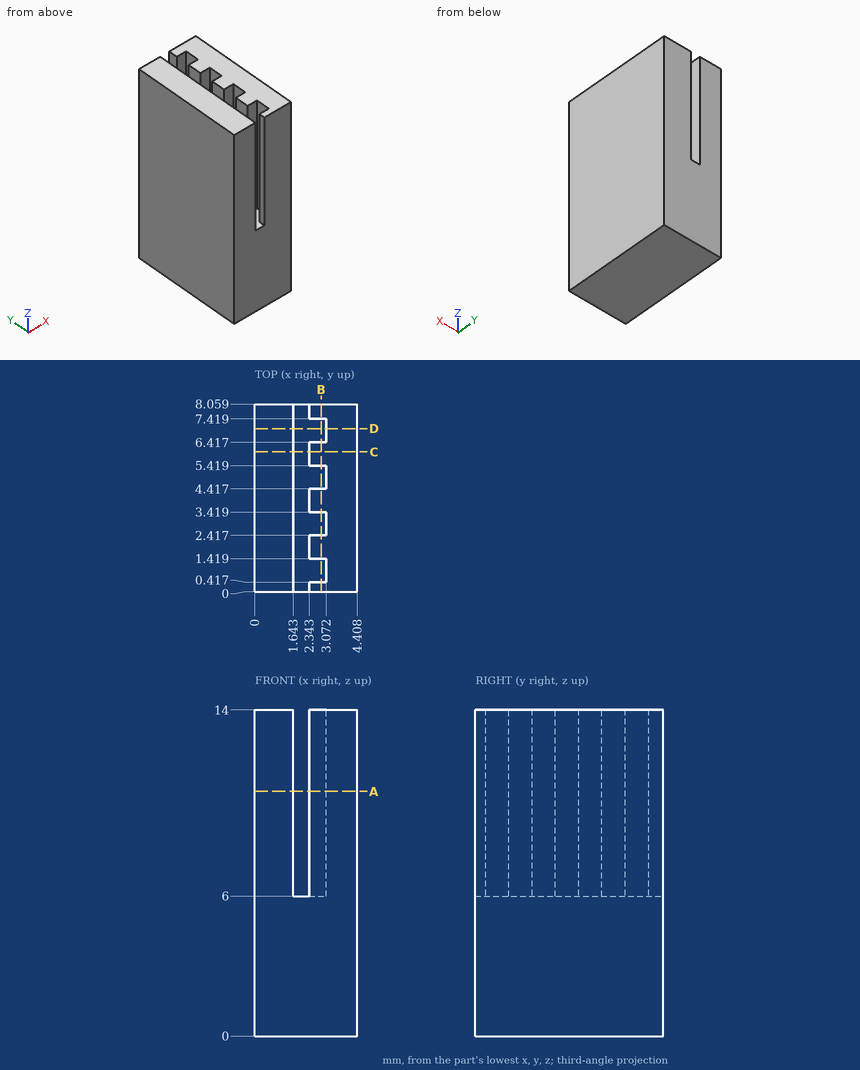
Geometry check sheet. Reference: drawing and pictorial views, mm from the part's lowest x, y, z. Round coordinates to 2 decimals unless told otherwise and drop trailing zeros. Write each loop counter-clockwise with the first axis right and the second up, starting at its lowest first coordinate (ties: lowest second). Pieces come first, ordered by that corner, then holes. Notation, with made-up numbers: (-19.5, 77) -> (12.5, 77) arc R24 ccw to (12.5, 114) -> close; hole circle Ø8 at (-18.75, -36.75). An arc over 180 degrees is marked (long way). Put each result on its own line as item: value.
1) Cross-section at D-D, the plane y = 7. Enter the section's corners in (x, z).
Recorded:
outline: (0, 0) -> (4.41, 0) -> (4.41, 14) -> (3.07, 14) -> (3.07, 6) -> (1.64, 6) -> (1.64, 14) -> (0, 14) -> close
2) Cross-section at B-B, the plane x = 2.85. Enter the section's corners in (y, z).
Recorded:
outline: (0, 0) -> (8.06, 0) -> (8.06, 14) -> (7.42, 14) -> (7.42, 6) -> (6.42, 6) -> (6.42, 14) -> (5.42, 14) -> (5.42, 6) -> (4.42, 6) -> (4.42, 14) -> (3.42, 14) -> (3.42, 6) -> (2.42, 6) -> (2.42, 14) -> (1.42, 14) -> (1.42, 6) -> (0.42, 6) -> (0.42, 14) -> (0, 14) -> close
3) Cross-section at A-A, the plane z = 10.5. Enter the section's corners in (x, y).
Recorded:
outline: (0, 0) -> (1.64, 0) -> (1.64, 8.06) -> (0, 8.06) -> close; (2.34, 0) -> (4.41, 0) -> (4.41, 8.06) -> (2.34, 8.06) -> (2.34, 7.42) -> (3.07, 7.42) -> (3.07, 6.42) -> (2.34, 6.42) -> (2.34, 5.42) -> (3.07, 5.42) -> (3.07, 4.42) -> (2.34, 4.42) -> (2.34, 3.42) -> (3.07, 3.42) -> (3.07, 2.42) -> (2.34, 2.42) -> (2.34, 1.42) -> (3.07, 1.42) -> (3.07, 0.42) -> (2.34, 0.42) -> close
4) Depth check by flat-ended pin: P1, Ø1.1, axis at y = 3, z = 10, coming from the -X side. Enter the tip coordinate at first touch or a pass-through.
Recorded:
P1: stops at x = 0
5) Thickness scan on probe 1 along X at (y, z) = (2, 12.75); probe 2 along X at (y, z) = (3, 9.5); probe 3 along Z at (x, y) = (1.8, 7). Record the ranges inside material, lowest first. Write a range as from..to.
Recorded:
probe 1: x = 0..1.64, 2.34..4.41
probe 2: x = 0..1.64, 3.07..4.41
probe 3: z = 0..6
6) Cross-section at C-C, the plane y = 6. Enter the section's corners in (x, z).
Recorded:
outline: (0, 0) -> (4.41, 0) -> (4.41, 14) -> (2.34, 14) -> (2.34, 6) -> (1.64, 6) -> (1.64, 14) -> (0, 14) -> close
